```python
from build123d import *

# Parameters (mm, degrees)
SKETCH1_W                       = 65
SKETCH1_H                       = 30
SKETCH1_W_2                     = 5
SKETCH1_H_2                     = 10
BOSS_EXTRUDE1_DEPTH             = 5
SKETCH1_4_W                     = 5
SKETCH1_4_H                     = 10
BOSS_EXTRUDE2_DEPTH             = 15
SKETCH2_R                       = 3
SKETCH2_R_2                     = 2.5
BOSS_EXTRUDE3_DEPTH             = 1
BOSS_EXTRUDE4_START             = 1
SKETCH3_R                       = 3
SKETCH3_R_2                     = 2.5
BOSS_EXTRUDE4_DEPTH             = 1
BOSS_EXTRUDE5_REACH             = 56.314
BOSS_EXTRUDE5_DIRECTION_2_REACH = 56.314
CUT_EXTRUDE2_DEPTH              = 35
SKETCH5_R                       = 1.75
CUT_EXTRUDE3_DEPTH              = 47.703854231
SKETCH7_R                       = 1
CUT_EXTRUDE5_DEPTH              = 4.5
SKETCH10_W                      = 10
SKETCH10_H                      = 15
BOSS_EXTRUDE7_DEPTH             = 20
CUT_EXTRUDE8_DEPTH              = 10


with BuildPart() as part:
    # Sketch1 → Boss-Extrude1 (new body)
    with BuildSketch(Plane(origin=(0, 0, 0), x_dir=(1, 0, 0), z_dir=(0, 1, 0))):
        Rectangle(SKETCH1_W, SKETCH1_H)
        with Locations((20, 5)):
            Rectangle(SKETCH1_W_2, SKETCH1_H_2, mode=Mode.SUBTRACT)
        with Locations((-20, 5)):
            Rectangle(SKETCH1_W_2, SKETCH1_H_2, mode=Mode.SUBTRACT)
    extrude(amount=BOSS_EXTRUDE1_DEPTH)

    # Sketch1<4> → Boss-Extrude2 (add)
    with BuildSketch(Plane(origin=(0, 0, 0), x_dir=(1, 0, 0), z_dir=(0, 1, 0))):
        with Locations((20, 5)):
            Rectangle(SKETCH1_4_W, SKETCH1_4_H)
        with Locations((-20, 5)):
            Rectangle(SKETCH1_4_W, SKETCH1_4_H)
    extrude(amount=BOSS_EXTRUDE2_DEPTH)

    # Sketch2 → Boss-Extrude3 (add)
    with BuildSketch(Plane(origin=(-17.5, 0, 0), x_dir=(0, 0, -1), z_dir=(1, 0, 0))):
        with Locations((5, 10)):
            Circle(SKETCH2_R)
        with Locations((5, 10)):
            Circle(SKETCH2_R_2, mode=Mode.SUBTRACT)
    extrude(amount=BOSS_EXTRUDE3_DEPTH)

    # Sketch3 → Boss-Extrude4 (add)
    with BuildSketch(Plane.ZY.offset(-17.5).offset(BOSS_EXTRUDE4_START)):
        with Locations(Location((-5, 10, 0), (0, 0, 180))):
            Circle(SKETCH3_R)
        with Locations(Location((-5, 10, 0), (0, 0, 180))):
            Circle(SKETCH3_R_2, mode=Mode.SUBTRACT)
    extrude(amount=-BOSS_EXTRUDE4_DEPTH)

    # Boss-Extrude5: up to this face of the body (flat: up to its plane)
    boss_extrude5_end = Plane(part.part.faces().sort_by_distance((22.5, 10, -5))[0])
    # Sketch4 → Boss-Extrude5 (add, up to the picked face)
    with BuildSketch(Plane(origin=(-17.5, 0, 0), x_dir=(0, 0, -1), z_dir=(1, 0, 0)), mode=Mode.PRIVATE) as boss_extrude5_sk1:
        Polygon((10.15, 5.5), (10.65, 5.5), (10.65, 3.5), (-0.65, 3.5), (-0.65, 5.5), (-0.15, 5.5), (-0.15, 4), (10.15, 4), align=None)
    boss_extrude5_tool1 = split(extrude(boss_extrude5_sk1.sketch, amount=BOSS_EXTRUDE5_REACH, mode=Mode.PRIVATE), bisect_by=boss_extrude5_end, keep=Keep.BOTH, mode=Mode.PRIVATE)
    add(boss_extrude5_tool1.solids().sort_by(Axis((-17.5, 3.95979, -5), (1, 0, 0)))[0])

    # Boss-Extrude5 direction 2: up to this face of the body (flat: up to its plane)
    boss_extrude5_direction_2_end = Plane(part.part.faces().sort_by_distance((-22.5, 10, -5))[0])
    # Sketch4 → Boss-Extrude5 direction 2 (add, up to the picked face)
    with BuildSketch(Plane(origin=(-17.5, 0, 0), x_dir=(0, 0, -1), z_dir=(1, 0, 0)), mode=Mode.PRIVATE) as boss_extrude5_direction_2_sk1:
        Polygon((10.15, 5.5), (10.65, 5.5), (10.65, 3.5), (-0.65, 3.5), (-0.65, 5.5), (-0.15, 5.5), (-0.15, 4), (10.15, 4), align=None)
    boss_extrude5_direction_2_tool1 = split(extrude(boss_extrude5_direction_2_sk1.sketch, amount=-BOSS_EXTRUDE5_DIRECTION_2_REACH, mode=Mode.PRIVATE), bisect_by=boss_extrude5_direction_2_end, keep=Keep.BOTH, mode=Mode.PRIVATE)
    add(boss_extrude5_direction_2_tool1.solids().sort_by(Axis((-17.5, 3.95979, -5), (-1, 0, 0)))[0])

    # Sketch4<5> → Cut-Extrude2 (cut)
    with BuildSketch(Plane(origin=(-17.5, 0, 0), x_dir=(0, 0, -1), z_dir=(1, 0, 0))):
        Polygon((0, 5.5), (-0.15, 5.5), (-0.15, 4), (10.15, 4), (10.15, 5.5), (10, 5.5), (10, 5), (0, 5), align=None)
    extrude(amount=CUT_EXTRUDE2_DEPTH, mode=Mode.SUBTRACT)

    # Sketch5 → Cut-Extrude3 (cut, through all)
    with BuildSketch(Plane.XY.offset(15)):
        with Locations((-27.5, 2.5)):
            Circle(SKETCH5_R)
    cut_extrude3 = extrude(amount=-CUT_EXTRUDE3_DEPTH, mode=Mode.SUBTRACT)

    # Mirror1: Cut-Extrude3 across plane
    add(cut_extrude3.mirror(Plane(origin=(0, 0, 0), x_dir=(0, 0, 1), z_dir=(1, 0, 0))), mode=Mode.SUBTRACT)

    # Sketch7 → Cut-Extrude5 (cut)
    with BuildSketch(Plane(origin=(0, 5, 0), x_dir=(1, 0, 0), z_dir=(0, 1, 0))):
        with Locations(Location((0, -10, 0), (0, 0, 270))):
            Circle(SKETCH7_R)
        with Locations(Location((0, -5, 0), (0, 0, 270))):
            Circle(SKETCH7_R)
    extrude(amount=-CUT_EXTRUDE5_DEPTH, mode=Mode.SUBTRACT)

    # Sketch10 → Boss-Extrude7 (add)
    with BuildSketch(Plane(origin=(0, 5, 0), x_dir=(1, 0, 0), z_dir=(0, 1, 0))):
        with Locations((0, -7.5)):
            Rectangle(SKETCH10_W, SKETCH10_H)
    extrude(amount=-BOSS_EXTRUDE7_DEPTH)

    # Sketch11 → Cut-Extrude8 (cut)
    with BuildSketch(Plane.XY.offset(15)):
        with BuildLine():
            ThreePointArc((-0.5, -4.031373033), (-4, -8), (-0.5, -11.968626967))
            Line((-0.5, -11.968626967), (-0.5, -4.031373033))
        make_face()
        with BuildLine():
            Line((0.5, -4.031373033), (0.5, -11.968626967))
            ThreePointArc((0.5, -11.968626967), (3, -10.645751311), (4, -8))
            ThreePointArc((4, -8), (3, -5.354248689), (0.5, -4.031373033))
        make_face()
    extrude(amount=-CUT_EXTRUDE8_DEPTH, mode=Mode.SUBTRACT)


solid = part.part
```
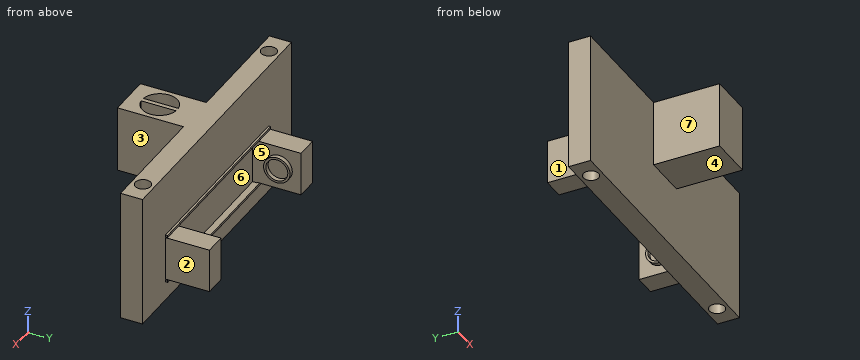
Check sheet for the modelled part. Datum: model origin and axes. Units: mm. Face numbers are marked on the shaded views. A direction names the side the tool comes from. Round coordinates to 2 decimals unless told otherwise and drop trailing zeros. Order: outer loops, then holes, each group sorted by start corner. A loop starts at its lowest first (then second) coordinate and runs counter-clockwise, first axis right, second up.
1) Tool access check on the marked faces 1, 2 and 3. Record the directions out of +Z, -Z, +X, -X, +Y, -Y that give a thin tool (end or side, any length) a straight path to the whole face; none if there is none.
2) Mould release check, pull along X, two halves, no side actions. Record for the marked faces 4, 5, 6 and 7: +X half, -X half, draft (parallel to the pull), parting line (faces both ways), or undercut.
3) Section check B-B (z = -5). Give the number of separate pieces and of enclosed holes in the cut face, and give its area (3 significant figures).
4) Section check D-D (x = -27.5). Record the boundary of the cut face in (y, z), and give its area (3 significant figures).
5) Section check C-C (y = 2.5). Record the boundary of the cut face in (x, z), and give its area (3 significant figures).
6) Scan lines: line 1 (Y direction, x = 16.85, z = -5); line 2 (Y direction, x = 27.5, z = -5.5); line 3 (Z direction, x = 17.1, y = 10). Record each from-to range of solid material in increasing order.
7) Section check A-A (y = 10). Record the boundary of the cut face in (x, z), and give its area (3 significant figures).
8) Go/stop test with flat-tipped pins: pin 1 Ø6.5 at (y, z) = (9.5, -4) entering from +X; pin 2 Ø1.5 at (x, y) = (-19.5, 8.5) entering from +Z; pin 3 Ø1.8 at (x, y) = (1.5, -10) entering from +Z; pin 4 Ø16.5 at (y, z) = (-7, 6) entering from -X. Record where each tip stops, or that it passes through.
Result:
1. face 1: +Z, -Z, -X, +Y
1. face 2: +Z, -Z, +X, +Y
1. face 3: +Z, -Z, +X, -Y
2. face 4: draft
2. face 5: undercut
2. face 6: undercut
2. face 7: -X half
3. separate pieces: 1
3. enclosed holes: 2
3. area: 373 mm2
4. outline: (0, -15) - (0.75, -15) - (0.75, 15) - (0, 15) - close; (4.25, -15) - (5, -15) - (5, 15) - (4.25, 15) - close
4. area: 45.0 mm2
5. outline: (-32.5, -15) - (-29.25, -15) - (-29.25, 15) - (-32.5, 15) - close; (-25.75, -15) - (25.75, -15) - (25.75, 15) - (-25.75, 15) - close; (29.25, -15) - (32.5, -15) - (32.5, 15) - (29.25, 15) - close
5. area: 1,740 mm2
6. line 1: y = 0 to 4, 7 to 7.5, 12.5 to 13
6. line 2: y = 0 to 0.75, 4.25 to 5
6. line 3: z = -8 to -7.5, -2.5 to -2
7. outline: (-22.5, -10) - (-17.5, -10) - (-17.5, -8) - (-16.5, -8) - (-16.5, -7.5) - (-17.5, -7.5) - (-17.5, -2.5) - (-16.5, -2.5) - (-16.5, -2) - (-17.5, -2) - (-17.5, 0) - (-22.5, 0) - close; (16.5, -8) - (17.5, -8) - (17.5, -10) - (22.5, -10) - (22.5, 0) - (17.5, 0) - (17.5, -2) - (16.5, -2) - (16.5, -2.5) - (17.5, -2.5) - (17.5, -7.5) - (16.5, -7.5) - close
7. area: 102 mm2
8. pin 1: stops at x = 22.5
8. pin 2: stops at z = 0
8. pin 3: stops at z = 5
8. pin 4: stops at x = -32.5
